Input: part model. Units: mm. Frame: model coordinates. A direction names the side the tool comes from. Round coordinates to 2 decimals unless told otherwise and drop trailing zeros. Order: outer loops, then holes, each group sorted by start corner. A loop starts at its lowest first (then second) coordinate and runs counter-clockwise, first axis right, second up. Notation, with made-up numbers: (-9, 86.5) -> (49, 86.5) arc R23 ccw to (49, 123.5) -> close; hole circle Ø5 at (-29, 45). An arc over 180 degrees is marked (long way). Use a Markdown table: item, result.
from build123d import *

# Parameters (mm, degrees)
RESSALTO_EXTRUS_O1_DEPTH   = 6.5
CORTE_EXTRUS_O1_DEPTH      = 34.71775564
CORTE_EXTRUS_O2_START      = -6.5
CORTE_EXTRUS_O2_DEPTH      = 1.5
ESBO_O5_R                  = 1.4
CORTE_EXTRUS_O3_DEPTH      = 47.75
CORTE_EXTRUS_O3_DEPTH_BACK = 6


with BuildPart() as part:
    # Esboço1 → Ressalto-extrusão1 (new body, symmetric)
    with BuildSketch(Plane(origin=(0, 0, 0), x_dir=(1, 0, 0), z_dir=(0, 1, 0))):
        with BuildLine():
            Line((0, 51.75), (18.140349372, 51.75))
            ThreePointArc((18.140349372, 51.75), (22.467809892, 50.765158648), (25.942897998, 48.004617089))
            ThreePointArc((25.942897998, 48.004617089), (33.71775564, 25.875), (25.942897998, 3.745382911))
            ThreePointArc((25.942897998, 3.745382911), (22.467809892, 0.984841352), (18.140349372, 0))
            Line((18.140349372, 0), (0, 0))
            Line((0, 0), (0, 5))
            Line((0, 5), (18.140349372, 5))
            ThreePointArc((18.140349372, 5), (20.304079632, 5.492420676), (22.041623685, 6.872691455))
            ThreePointArc((22.041623685, 6.872691455), (28.71775564, 25.875), (22.041623685, 44.877308545))
            ThreePointArc((22.041623685, 44.877308545), (20.304079632, 46.257579324), (18.140349372, 46.75))
            Line((18.140349372, 46.75), (0, 46.75))
            Line((0, 46.75), (0, 51.75))
        make_face()
    extrude(amount=RESSALTO_EXTRUS_O1_DEPTH, both=True)

    # Esboço2 → Corte-extrusão1 (cut, through all)
    with BuildSketch(Plane.ZY):
        with BuildLine():
            Line((-44.75, 2.6), (-7, 2.6))
            ThreePointArc((-7, 2.6), (-5.6, 4), (-7, 5.4))
            Line((-7, 5.4), (-44.75, 5.4))
            ThreePointArc((-44.75, 5.4), (-46.15, 4), (-44.75, 2.6))
        make_face()
        with BuildLine():
            Line((-44.75, -5.4), (-7, -5.4))
            ThreePointArc((-7, -5.4), (-5.6, -4), (-7, -2.6))
            Line((-7, -2.6), (-44.75, -2.6))
            ThreePointArc((-44.75, -2.6), (-46.15, -4), (-44.75, -5.4))
        make_face()
    extrude(amount=-CORTE_EXTRUS_O1_DEPTH, mode=Mode.SUBTRACT)

    # Esboço4 → Corte-extrusão2 (cut, symmetric)
    with BuildSketch(Plane(origin=(0, 6.5, 0), x_dir=(1, 0, 0), z_dir=(0, 1, 0)).offset(CORTE_EXTRUS_O2_START)):
        with BuildLine():
            Line((8.48, 35.63), (13.203313178, 51.75))
            Line((13.203313178, 51.75), (33.71775564, 51.75))
            Line((33.71775564, 51.75), (33.71775564, 0))
            Line((33.71775564, 0), (17.161678374, 0))
            Line((17.161678374, 0), (11.37, 10.3))
            ThreePointArc((11.37, 10.3), (7.366682193, 22.673111391), (8.48, 35.63))
        make_face()
    extrude(amount=CORTE_EXTRUS_O2_DEPTH, both=True, mode=Mode.SUBTRACT)

    # Esboço5 → Corte-extrusão3 (cut, two sides)
    with BuildSketch(Plane.XY.offset(-46.75)) as corte_extrus_o3_sk:
        with Locations((2.25, 4.25)):
            Circle(ESBO_O5_R)
        with Locations((2.25, -4.25)):
            Circle(ESBO_O5_R)
    extrude(amount=CORTE_EXTRUS_O3_DEPTH, mode=Mode.SUBTRACT)
    extrude(corte_extrus_o3_sk.sketch, amount=-CORTE_EXTRUS_O3_DEPTH_BACK, mode=Mode.SUBTRACT)


solid = part.part
1) Pull-direction query (X, two-part tool) for faces 1 (the cylindrical face through (24.33, 4.03, -46.15)), 2 (the cylindrical face through (3.54, 3.71, -49.22)), 3 (the cylindrical face through (19.82, 4.04, -5.29)); classes: +X half, -X half, draft (parallel to the pull), parting line (faces both ways), or undercut.
Results found:
| item | result |
|---|---|
| face 1 | draft |
| face 2 | undercut |
| face 3 | -X half |
2) Line query: L1, parallel to Y at x = 2.25, z = -1.05; L2, parallel to Y at x = 29, z = -20.5; L3, parallel to Z at x = 16.5, y = 1.75. Output: solid intervals per line, ascending. Write a range as [from, to].
Results found:
| item | result |
|---|---|
| L1 | y = [-6.5, -5.65], [-2.85, 2.85], [5.65, 6.5] |
| L2 | y = [-6.5, -5.4], [-2.6, -1.5], [1.5, 2.6], [5.4, 6.5] |
| L3 | z = [-51.75, -46.75], [-5, 0] |
3) Set-up query: faces 4 (the cylindrical face through (19.875, -3.965, -46.439)), 5 (the flat face through (15.776, 0.021, -2.465)), 6 (the flat face through (29, 5.4, -26)), 7 (the flat face through (12.46, 0.02, -49.22)). Return all of +Z, -Z, +X, -X, +Y, -Y with unobstructed straight access to the full face (end or side cutting, diameter ignored); none if empty.
Results found:
| item | result |
|---|---|
| face 4 | -X, +Y, -Y |
| face 5 | -Z, +X |
| face 6 | +X, -X |
| face 7 | +X |
4) Cut plane B-B on x = 2.25. Return loops of the section in (y, z), and give its area (3 significant figures).
Results found:
| item | result |
|---|---|
| outline | (-6.5, -51.75) -> (-5.65, -51.75) -> (-5.65, -46.75) -> (-6.5, -46.75) -> close; (-6.5, -5) -> (-5.65, -5) -> (-5.65, 0) -> (-6.5, 0) -> close; (-2.85, -51.75) -> (2.85, -51.75) -> (2.85, -46.75) -> (-2.85, -46.75) -> close; (-2.85, -5) -> (2.85, -5) -> (2.85, 0) -> (-2.85, 0) -> close; (5.65, -51.75) -> (6.5, -51.75) -> (6.5, -46.75) -> (5.65, -46.75) -> close; (5.65, -5) -> (6.5, -5) -> (6.5, 0) -> (5.65, 0) -> close |
| area | 74.0 mm² |
5) Cut plane A-A on y = 0. Return loops of the section in (x, z).
Results found:
| item | result |
|---|---|
| outline | (0, -51.75) -> (13.2, -51.75) -> (11.74, -46.75) -> (0, -46.75) -> close; (0, -5) -> (14.35, -5) -> (17.16, 0) -> (0, 0) -> close |
6) Pin query (flat end, axial travel): pin 1 Ø3 at (y, z) = (4.5, -21) entering from +X; pin 2 Ø12 at (x, z) = (9, -39) entering from -Y; pin 3 Ø4 at (y, z) = (5, -15.5) entering from +X. Return the tip coordinate at first contact, or that it passes through.
Results found:
| item | result |
|---|---|
| pin 1 | stops at x = 33.53 |
| pin 2 | passes through |
| pin 3 | stops at x = 32.7 |
7) Cut plane D-D on x = 30. Return loops of the section in (y, z), and give its area (3 significant figures).
Results found:
| item | result |
|---|---|
| outline | (-6.5, -41.66) -> (-5.4, -41.66) -> (-5.4, -10.09) -> (-6.5, -10.09) -> close; (-2.6, -41.66) -> (-1.5, -41.66) -> (-1.5, -10.09) -> (-2.6, -10.09) -> close; (1.5, -41.66) -> (2.6, -41.66) -> (2.6, -10.09) -> (1.5, -10.09) -> close; (5.4, -41.66) -> (6.5, -41.66) -> (6.5, -10.09) -> (5.4, -10.09) -> close |
| area | 139 mm² |
8) Cut plane C-C on z = -13.5. Return loops of the section in (x, y).
Results found:
| item | result |
|---|---|
| outline | (26.08, -6.5) -> (31.48, -6.5) -> (31.48, -5.4) -> (26.08, -5.4) -> close; (26.08, -2.6) -> (31.48, -2.6) -> (31.48, -1.5) -> (26.08, -1.5) -> close; (26.08, 1.5) -> (31.48, 1.5) -> (31.48, 2.6) -> (26.08, 2.6) -> close; (26.08, 5.4) -> (31.48, 5.4) -> (31.48, 6.5) -> (26.08, 6.5) -> close |
